```python
from build123d import *

# Parameters (mm, degrees)
SKETCH3_R           = 6.096
BOSS_EXTRUDE1_DEPTH = 7.874


with BuildPart() as part:
    # Sketch1 → Base-Revolve (revolve)
    with BuildSketch(Plane.XY):
        with BuildLine():
            Line((6.096, 0), (6.096, 14.732))
            Line((6.096, 14.732), (4.826, 16.002))
            Line((4.826, 16.002), (2.286, 16.002))
            Line((2.286, 16.002), (2.286, 15.494))
            Line((2.286, 15.494), (1.778, 15.494))
            Line((1.778, 15.494), (1.778, 13.462))
            ThreePointArc((1.778, 13.462), (3.53667068, 11.915498853), (4.191, 9.666845589))
            Line((4.191, 9.666845589), (4.191, 0))
            Line((4.191, 0), (6.096, 0))
        make_face()
    revolve(axis=Axis((0, 0, 0), (0, 1, 0)))

    # Sketch3 → Boss-Extrude1 (add)
    with BuildSketch(Plane(origin=(0, 12.954, 0), x_dir=(-1, 0, 0), z_dir=(0, 1, 0))):
        Polygon((3.739497694, -6.477), (-3.739497694, -6.477), (-7.478995387, 0), (-3.739497694, 6.477), (3.739497694, 6.477), (7.478995387, 0), align=None)
        Circle(SKETCH3_R, mode=Mode.SUBTRACT)
    extrude(amount=-BOSS_EXTRUDE1_DEPTH)

    # Sketch4 → Cut-Revolve1 (revolve, cut)
    with BuildSketch(Plane.XY):
        with BuildLine():
            Line((7.478995387, 12.954), (6.096, 12.954))
            ThreePointArc((6.096, 12.954), (6.793780049, 12.676772421), (7.478995387, 12.3698))
            Line((7.478995387, 12.3698), (7.478995387, 12.954))
        make_face()
    cut_revolve1 = revolve(axis=Axis((0, 0, 0), (0, 1, 0)), mode=Mode.SUBTRACT)

    # Mirror1: Cut-Revolve1 across plane
    add(cut_revolve1.mirror(Plane.ZX.offset(9.017)), mode=Mode.SUBTRACT)


solid = part.part
```
The listing builds one solid part. Answer for the finished solid, in the listing's coordinates (mm). A direction names the side the tool comes from. Give positions to 0.01 mm unless a question says otherwise; leave off trailing zeros. Loops run counter-clockwise (first coordinate to the right, second up) from the corner with the lowest first, then second, coordinate; pieces in that order, holes last. Notation, with made-up numbers: (86, 85) - (110, 85) arc R24 ccw to (110, 112) - close; hole circle Ø6 at (38, 79). An arc over 180 degrees is marked (long way). Return JSON: item names as keys, results as strings. Group by question number.
1. Straight lines are drawn through the part: line 1 (Z direction, x = 0, y = 2.25); line 2 (Z direction, x = 0, y = 14.05); line 3 (X direction, y = 11, z = 1.75). For each, find the intervals that lie inside material, in ascending order. Write a range as [from, to].
2. Which of the six approach directions +Z, -Z, +X, -X, +Y, -Y give full straight-line access (tool end or side, diameter ignored) to faces 4 (the cylindrical face through (3.997, 4.766, -1.259)), 5 (the cylindrical face through (-0.794, 13.855, -6.044)), 6 (the flat face through (1.44, 0, -4.15))?
3. Find section A-A (y = 13.75). Write down the section's boundary in (x, z).
4. Given pin 1 Ø2 at (y, z) = (9, 0.5) entering from -X; pin 2 Ø5 at (x, z) = (0, 0) entering from -Y; pin 3 Ø2 at (x, z) = (5.5, -2) entering from +Y, each flat-ended and moving along its own axis, determine where each tip first touches the part or whether it passes through.
5. Determine the mould class of faces 1 (the cylindrical face through (-0.385, 14.464, 1.736)), 2 (the flat face through (-5.635, 9.07, -3.193)), 3 (the cylindrical face through (-0.794, 2.576, -6.044)) for opening direction X: pulls with the +X half, pulls with the -X half, needs draft (parallel to the pull), parting line crosses it, or undercut.
Verdict:
{
 "1": {"line 1": "z = [-6.1, -4.19], [4.19, 6.1]", "line 2": "z = [-6.1, -1.78], [1.78, 6.1]", "line 3": "x = [-6.47, -3.57], [3.57, 6.47]"},
 "2": {"face 4": "-Y", "face 5": "+Y", "face 6": "+Z, -Z, +X, -X, -Y"},
 "3": {"outline": "circle Ø12.19 at (0, 0); hole circle Ø3.56 at (0, 0)"},
 "4": {"pin 1": "stops at x = -7.48", "pin 2": "stops at y = 13.03", "pin 3": "stops at y = 15.98"},
 "5": {"face 1": "undercut", "face 2": "pulls with the -X half", "face 3": "parting line crosses it"}
}
